Check sheet for the modelled part. Datum: model origin and axes. Units: mm. A direction names the side the tool comes from. Round coordinates to 2 decimals unless told otherwise and drop trailing zeros. Write each loop counter-clockwise with the first axis right and the second up, starting at its lowest first coordinate (ties: lowest second). Pieces come first, ordered by that corner, then holes. Notation, with made-up numbers: (48, -4.75) -> (90, -4.75) arc R32 cw to (90, 25.25) -> close; hole circle Ø5 at (-25.75, 62.25). An arc over 180 degrees is marked (long way). One line per item, written item: value.
from build123d import *

# Parameters (mm, degrees)
BOSS_EXTRUDE2_DEPTH = 3
MOD_BAT_W           = 29
MOD_BAT_H           = 18
CUT_MOD_BAT_DEPTH   = 1
PICO_W              = 52
PICO_H              = 22
CUT_PICO_DEPTH      = 2
SD_CARD_W           = 19
SD_CARD_H           = 19
CUT_SD_CARD_DEPTH   = 1
SD_PIN_W            = 3
SD_PIN_H            = 19
CUT_SD_PIN_DEPTH    = 2
ACELEROMETRO1_W     = 28
ACELEROMETRO1_H     = 16
CUT_ACL1_DEPTH      = 1
STEP_UP_W           = 19
STEP_UP_H           = 37
CUT_STEPUP_DEPTH    = 1
ACELEROMETRO2_W     = 28
ACELEROMETRO2_H     = 16
CUT_ACL2_DEPTH      = 1
SKETCH10_W          = 28
SKETCH10_H          = 4
CUT_ACL1_PIN_DEPTH  = 2
SKETCH10_3_W        = 28
SKETCH10_3_H        = 4
CUT_ACL2_PIN_DEPTH  = 2
SKETCH11_W          = 3
SKETCH11_H          = 40
BOSS_EXTRUDE3_DEPTH = 40
SKETCH12_W          = 20
SKETCH12_H          = 40
CUT_EXTRUDE15_DEPTH = 1


with BuildPart() as part:
    # Sketch7 → Boss-Extrude2 (new body)
    with BuildSketch(Plane(origin=(0, 0, 0), x_dir=(1, 0, 0), z_dir=(0, 1, 0))):
        Polygon((-65, 20), (-102, 20), (-102, -20), (-79, -20), (-79, -35), (-24, -35), (-24, -38), (0, -38), (0, 37), (-33, 37), (-33, 35), (-65, 35), align=None)
    extrude(amount=-BOSS_EXTRUDE2_DEPTH)

    # Mod. Bat → Cut-mod Bat (cut)
    with BuildSketch(Plane(origin=(0, 0, 0), x_dir=(1, 0, 0), z_dir=(0, 1, 0))):
        with Locations((-14.5, 24)):
            Rectangle(MOD_BAT_W, MOD_BAT_H)
    extrude(amount=-CUT_MOD_BAT_DEPTH, mode=Mode.SUBTRACT)

    # Pico → Cut-Pico (cut)
    with BuildSketch(Plane(origin=(0, 0, 0), x_dir=(1, 0, 0), z_dir=(0, 1, 0))):
        with Locations((-26, 0)):
            Rectangle(PICO_W, PICO_H)
    extrude(amount=-CUT_PICO_DEPTH, mode=Mode.SUBTRACT)

    # SD Card → Cut-SD Card (cut)
    with BuildSketch(Plane(origin=(0, 0, 0), x_dir=(1, 0, 0), z_dir=(0, 1, 0))):
        with Locations((-9.5, -24.5)):
            Rectangle(SD_CARD_W, SD_CARD_H)
    extrude(amount=-CUT_SD_CARD_DEPTH, mode=Mode.SUBTRACT)

    # SD Pin → Cut-SD Pin (cut)
    with BuildSketch(Plane(origin=(0, 0, 0), x_dir=(1, 0, 0), z_dir=(0, 1, 0))):
        with Locations((-17.5, -24.5)):
            Rectangle(SD_PIN_W, SD_PIN_H)
    extrude(amount=-CUT_SD_PIN_DEPTH, mode=Mode.SUBTRACT)

    # Acelerometro1 → Cut-Acl1 (cut)
    with BuildSketch(Plane(origin=(0, 0, 0), x_dir=(1, 0, 0), z_dir=(0, 1, 0))):
        with Locations((-38, -23)):
            Rectangle(ACELEROMETRO1_W, ACELEROMETRO1_H)
    extrude(amount=-CUT_ACL1_DEPTH, mode=Mode.SUBTRACT)

    # step-up → Cut-StepUp (cut)
    with BuildSketch(Plane(origin=(0, 0, 0), x_dir=(1, 0, 0), z_dir=(0, 1, 0))):
        with Locations((-65.5, -12.5)):
            Rectangle(STEP_UP_W, STEP_UP_H)
    extrude(amount=-CUT_STEPUP_DEPTH, mode=Mode.SUBTRACT)

    # Acelerometro2 → Cut-Acl2 (cut)
    with BuildSketch(Plane(origin=(0, 0, 0), x_dir=(1, 0, 0), z_dir=(0, 1, 0))):
        with Locations((-47, 23)):
            Rectangle(ACELEROMETRO2_W, ACELEROMETRO2_H)
    extrude(amount=-CUT_ACL2_DEPTH, mode=Mode.SUBTRACT)

    # Sketch10 → Cut-Acl1 Pin (cut)
    with BuildSketch(Plane(origin=(0, 0, 0), x_dir=(1, 0, 0), z_dir=(0, 1, 0))):
        with Locations((-47, 17)):
            Rectangle(SKETCH10_W, SKETCH10_H)
    extrude(amount=-CUT_ACL1_PIN_DEPTH, mode=Mode.SUBTRACT)

    # Sketch10<3> → Cut-Acl2 Pin (cut)
    with BuildSketch(Plane(origin=(0, 0, 0), x_dir=(1, 0, 0), z_dir=(0, 1, 0))):
        with Locations((-38, -29)):
            Rectangle(SKETCH10_3_W, SKETCH10_3_H)
    extrude(amount=-CUT_ACL2_PIN_DEPTH, mode=Mode.SUBTRACT)

    # Sketch11 → Boss-Extrude3 (add)
    with BuildSketch(Plane(origin=(0, 0, 0), x_dir=(1, 0, 0), z_dir=(0, 1, 0))):
        with Locations((-100.5, 0)):
            Rectangle(SKETCH11_W, SKETCH11_H)
    extrude(amount=BOSS_EXTRUDE3_DEPTH)

    # Sketch12 → Cut-Extrude15 (cut)
    with BuildSketch(Plane(origin=(0, 0, 0), x_dir=(1, 0, 0), z_dir=(0, 1, 0))):
        with Locations((-89, 0)):
            Rectangle(SKETCH12_W, SKETCH12_H)
    extrude(amount=-CUT_EXTRUDE15_DEPTH, mode=Mode.SUBTRACT)


solid = part.part
Item 1: Sectioned sample at B-B on z = -22.5. Enter the section's corners in (x, y).
Answer:
outline: (-65, -3) -> (0, -3) -> (0, -1) -> (-29, -1) -> (-29, 0) -> (-33, 0) -> (-33, -1) -> (-61, -1) -> (-61, 0) -> (-65, 0) -> close
Item 2: Mould release check, pull along Z, two halves, no side actions. Record for faces 1 (the flat face through (-47, -2, -17)), 2 (the flat face through (-16, -1, -37)), 3 (the flat face through (-26, -2, 0)), 4 (the flat face through (-52, -3, 0)): pulls with the +Z half, pulls with the -Z half, needs draft (parallel to the pull), parting line crosses it, or undercut.
Answer:
face 1: undercut
face 2: pulls with the -Z half
face 3: undercut
face 4: needs draft
Item 3: Thickness scan on line 1 (X direction, y = 20, z = 0.5); line 2 (Y direction, x = -15, z = -17); line 3 (Y direction, x = -39, z = -4). Record the ranges inside material, lowest first.
Answer:
line 1: x = -102 to -99
line 2: y = -3 to -1
line 3: y = -3 to -2
Item 4: Tool access check on faces 5 (the flat face through (-49, -1, -35)), 6 (the flat face through (-66, -1, 12)), 7 (the flat face through (-89, -1, 0)), 8 (the flat face through (-15, -1, -24)). Record the directions out of +Z, -Z, +X, -X, +Y, -Y that give a thin tool (end or side, any length) a straight path to the whole face; none if there is none.
Answer:
face 5: -Z, -X, +Y, -Y
face 6: +Y
face 7: +Z, -Z, +Y
face 8: +X, +Y
Item 5: Sectioned sample at D-D on x = -69.5. Enter the section's corners in (y, z).
Answer:
outline: (-3, -20) -> (0, -20) -> (0, -6) -> (-1, -6) -> (-1, 31) -> (0, 31) -> (0, 35) -> (-3, 35) -> close
Item 6: Sectioned sample at C-C on y = 13.5. Enter the section's corners in (x, z).
Answer:
outline: (-102, -20) -> (-99, -20) -> (-99, 20) -> (-102, 20) -> close
Item 7: Sectioned sample at A-A on x = -12. Enter the section's corners in (y, z).
Answer:
outline: (-3, -37) -> (0, -37) -> (0, -33) -> (-1, -33) -> (-1, -15) -> (0, -15) -> (0, -11) -> (-2, -11) -> (-2, 11) -> (0, 11) -> (0, 15) -> (-1, 15) -> (-1, 34) -> (0, 34) -> (0, 38) -> (-3, 38) -> close
Item 8: Depth check by flat-ended pin: P1, Ø0.9, axis at x = -17.5, z = 20, coming from the +Y side; P2, Ø6, axis at y = 16, z = 23.5, coming from the -X side; P3, Ø12, axis at y = 11.5, z = 9, coming from the +X side; P4, Ø1.5, axis at y = -1, z = 36, coming from the -X side. Enter the tip coordinate at first touch or a pass-through.
Answer:
P1: stops at y = -2
P2: passes through
P3: stops at x = -99
P4: stops at x = -24
